Can you work these out from the model? Positions are in its coordinate system, mm. Face numbers are marked on the shaded views. A direction names the side the tool comes from. Give positions to 0.01 mm unless a question says otherwise; leave off trailing zeros. Write each loop counter-clockwise with the first axis right and the second up, starting at its lowest first coordinate (ties: lowest second). Pieces come first, ordered by that corner, then holes.
Autodesk Inventor part; units mm, degrees
ref_plane "Arbeitsebene1" through (-25, -20, 0) normal (0, -1, 0) x (1, 0, 0)
ref_plane "YZ Plane" through (0, 0, 0) normal (1, 0, 0) x (0, 1, 0)
ref_plane "XZ Plane" through (0, 0, 0) normal (0, 1, 0) x (-1, 0, 0)
sketch "Skizze1" plane through (0, 0, 0) normal (0, 0, 1) x (1, 0, 0)
  line L0 (-25, 25) -> (25, 25)
  line L1 (25, 25) -> (25, -25)
  line L2 (25, -25) -> (-25, -25)
  line L3 (-25, -25) -> (-25, 25)
  line L4 (-25, 25) -> (25, -25) construction
  line L5 (25, 25) -> (-25, -25) construction
  line L6 (20, 20) -> (23, 20) construction
  line L7 (-20, -20) -> (20, -20) construction
  line L8 (20, -20) -> (20, 20) construction
  line L9 (20, 20) -> (-20, 20) construction
  line L10 (-20, 20) -> (-20, -20) construction
  line L11 (-20, -20) -> (20, 20) construction
  line L12 (20, -20) -> (-20, 20) construction
  line L13 (-14, 19) -> (14, 19)
  line L14 (19, 14) -> (19, -14)
  line L15 (14, -19) -> (-14, -19)
  line L16 (-19, -14) -> (-19, 14)
  line L17 (-19, 19) -> (19, -19) construction
  line L18 (19, 19) -> (-19, -19) construction
  arc A0 (14, -19) -> (19, -14) centre (14, -14) ccw
  arc A1 (19, 14) -> (14, 19) centre (14, 14) ccw
  arc A2 (-14, 19) -> (-19, 14) centre (-14, 14) ccw
  arc A3 (-19, -14) -> (-14, -19) centre (-14, -14) ccw
  point P0 (0, 0)
  point P1 (0, 0)
  dimension "d2" = 50
  dimension "d3" = 50
  dimension "d273" = 40
  dimension "d274" = 40
  dimension "d275" = 38
  dimension "d276" = 38
  dimension "d277" = 5
extrude "Extrusion1" add sketch "Skizze1" along normal blind 5
ref_plane "Arbeitsebene1" through (-25, -20, 0) normal (0, -1, 0) x (1, 0, 0)
sketch "Skizze5" plane through (-25, -20, 0) normal (0, -1, 0) x (1, 0, 0)
  line L0 (50, 0) -> (0, 0)
  line L1 (0, 0) -> (0, 5)
  line L2 (5, -0.15) -> (5, 5.15)
  line L3 (5, 1) -> (7.1846, 1)
  line L4 (2.7, -1.6033) -> (2.7, 1.1838)
  line L5 (5, -1.6033) -> (5, -0.15)
  arc A0 (2.7, 3.8162) -> (4.1211, 0) centre (5, 2.5) ccw
  arc A1 (5, -0.15) -> (5, 5.15) centre (5, 2.5) ccw
  line L6 (7.1846, 1) -> (8.3346, -0.15)
  line L7 (8.3346, -0.15) -> (5, -0.15)
  line L8 (5, 2.5) -> (6.8859, 2.5)
  line L9 (7.1846, 4) -> (8.3346, 5.15)
  line L10 (8.3346, 5.15) -> (5, 5.15)
  point P0 (25, 0)
  point P1 (40, 8)
  point P2 (6.6949, -37.8745)
  dimension "d237" = 2.5
  dimension "d238" = 5
  dimension "d240" = 2.3
  dimension "d247" = 135
  dimension "d248" = 1.5
  dimension "d249" = 2.65
revolve "Umdrehung1" cut sketch "Skizze5" angle 360 about axis through (-20, -20, -0.15) along (0, 0, 1) contours L6 L7 A1 L0 | L0 A1 L6 | A1 L2 L0 | L0 L2 L3 A1 | L3 L2 A1 | A1 L10 L9
pattern_linear "Rechteckige Anordnung7" count 2 spacing 40 along (1, 0, 0) count 2 spacing 40 along (0, 1, 0) of "Umdrehung1"
sketch "Skizze16" plane through (0, 0, 0) normal (0, 0, -1) x (-1, 0, 0)
  line L0 (25, 25) -> (-25, 25)
  line L1 (-25, 25) -> (-25, -25)
  line L2 (-25, -25) -> (25, -25)
  line L3 (25, -25) -> (25, 25)
  circle A0 centre (0, 0) radius 25
  line L4 (-25, -25) -> (25, -25)
  line L5 (25, 25) -> (-25, 25)
  line L6 (25, 25) -> (25, -25)
  circle A1 centre (-20, 20) radius 3.1846
  circle A2 centre (20, 20) radius 3.1846
  circle A3 centre (20, -20) radius 3.1846
  circle A4 centre (-20, -20) radius 3.1846
  point P0 (0, -25)
  point P1 (-25, 0)
  point P2 (0, 25)
  point P3 (25, 0)
sketch "Skizze17" plane through (25, -15.5, 1) normal (-1, 0, 0) x (0, 0, 1)
  line L0 (-1, 40.5) -> (-1, -9.5)
  line L1 (-1, 40.5) -> (4, 40.5)
  line L2 (4, -9.5) -> (4, 40.5)
  line L3 (4, -9.5) -> (4, 40.5)
  line L4 (-1, -9.5) -> (4, -9.5)
  line L5 (-1, 40.5) -> (-1, -9.5)
  circle A0 centre (1.5, 26.5) radius 1.4
  circle A1 centre (1.5, 4.5) radius 1.4
  line L6 (-1, 40.5) -> (4, 40.5)
  line L7 (-1, -9.5) -> (4, -9.5)
  dimension "d241" = 2.8
  dimension "d242" = 2.8
  dimension "d243" = 14
  dimension "d1" = 14
  dimension "d253" = 2.5
  dimension "d254" = 2.5
extrude "Extrusion12" cut sketch "Skizze17" along normal blind 10 contours A0 | A1
sketch "Sketch24" plane through (0, 0, 0) normal (0, 0, -1) x (-1, 0, 0)
  circle A0 centre (20, -20) radius 3.1846
  circle A1 centre (-20, -20) radius 3.1846
  circle A2 centre (20, 20) radius 3.1846
  circle A3 centre (-20, 20) radius 3.1846
  line L0 (25, 25) -> (-25, 25)
  line L1 (-25, 25) -> (-25, -25)
  line L2 (-25, -25) -> (25, -25)
  line L3 (25, -25) -> (25, 25)
  circle A4 centre (0, 0) radius 12.0567
pattern_circular "Circular Pattern4" count 4 over 360 about axis through (0, 0, 0) along (0, 0, 1) of "Extrusion12"
equation "\"d2\" = d_part"
equation "\"d3\" = d_part"
equation "\"d_i\" = 40"
equation "\"d_o\" = 40"
equation "\"d_part\" = 50"
equation "\"d6\" = 0"
equation "\"d7\" = 0"
equation "\"d8\" = 0"
equation "\"d9\" = 0"
equation "\"d13\" = 0"
equation "\"d14\" = 0"
equation "\"d20\" = 0"
equation "\"d21\" = 0"
equation "\"d22\" = 0"
equation "\"d23\" = 0"
equation "\"d24\" = 0"
equation "\"d25\" = 3"
equation "\"d26\" = 0"
equation "\"d27\" = 0"
equation "\"d28\" = 0"
equation "\"d29\" = 0"
equation "\"d30\" = 0"
equation "\"d31\" = 0"
equation "\"d32\" = 0"
equation "\"d33\" = 0"
equation "\"d34\" = 0"
equation "\"d46\" = 0"
equation "\"d47\" = 0"
equation "\"d48\" = 0"
equation "\"d50\" = 0"
equation "\"d51\" = 0"
equation "\"d52\" = 0"
equation "\"d53\" = 0"
equation "\"d54\" = 0"
equation "\"d55\" = 0"
equation "\"d56\" = 0"
equation "\"d57\" = 0"
equation "\"d58\" = 0"
equation "\"d59\" = 0"
properties part number "10_Base_v2"
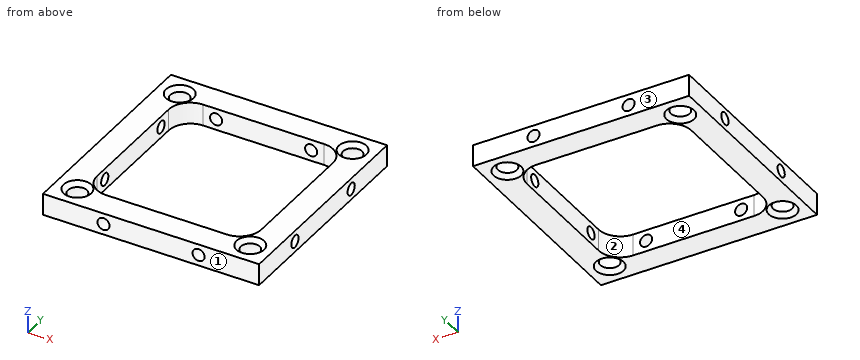
1) Suppose I cut it at B-B on x = -11. Write out the boundary of the cut face in (y, z).
Values follow:
outline: (-25, 0) - (-19, 0) - (-19, 1.1) - (-25, 1.1) - close; (-25, 3.9) - (-19, 3.9) - (-19, 5) - (-25, 5) - close; (19, 0) - (25, 0) - (25, 1.1) - (19, 1.1) - close; (19, 3.9) - (25, 3.9) - (25, 5) - (19, 5) - close
2) Suppose I cut it at A-A on y = 1. Write out the boundary of the cut face in (x, z), plus the area to 3 significant figures.
Values follow:
outline: (-25, 0) - (-19, 0) - (-19, 5) - (-25, 5) - close; (19, 0) - (25, 0) - (25, 5) - (19, 5) - close
area: 60.0 mm2
3) For pin 1 Ø2.5 at (x, z) = (-11, 2.5) entering from +Y, with a flat end and sliding along its axis, tell me the tip position at first contact or that it passes through.
Values follow:
pin 1: passes through
4) For the marked faces 3 and 4, which set-ups out of +Z, -Z, +X, -X, +Y, -Y let a thin tool reach every point of the face, with its end or its side?
Values follow:
face 3: +Z, -Z, +X, -X, +Y
face 4: +Z, -Z
5) If we mould it in two halves opening along X, with no side actions, what happens to the marked faces 1 and 2? For each: +X half, -X half, draft (parallel to the pull), parting line (faces both ways), or undercut.
Values follow:
face 1: draft
face 2: undercut
6) Please list where these lines run through material, in increasing order: L1, parallel to X at y = -20.5, z = 4.5; L2, parallel to Z at x = 11, y = -20.8; L3, parallel to Y at x = 14, z = 3.4.
Values follow:
L1: x = -25 to -22.64, -17.36 to 17.36, 22.64 to 25
L2: z = 0 to 1.1, 3.9 to 5
L3: y = -25 to -19, 19 to 25
